The model under review builds one solid part; all positions refer to its coordinate system, in mm. Coordinates: 2 decimals unless noted, no trailing zeros. Write each loop counter-clockwise with the first axis right and the second up, starting at its lowest first coordinate (ties: lowest second). Pieces come first, ordered by that corner, then holes.
```python
from build123d import *

# Parameters (mm, degrees)
SKETCH_1_W           = 111
SKETCH_1_H           = 96
EXTRUDE_1_DEPTH      = 3
SKETCH_2_R           = 1.6
CUT_EXTRUDE_1_DEPTH  = 74.438749989
SKETCH_3_R           = 2.6
CUT_EXTRUDE_2_DEPTH  = 74.438749989
SKETCH_4_R           = 1.6
CUT_EXTRUDE_3_DEPTH  = 74.438749989
SKETCH_8_R           = 2.6
CUT_EXTRUDE_10_DEPTH = 74.438749989
SKETCH_5_W           = 18
SKETCH_5_H           = 50
CUT_EXTRUDE_4_DEPTH  = 74.438749989
FILLET_1_R           = 4
CUT_EXTRUDE_8_DEPTH  = 74.438749989
FILLET_2_R           = 2.5
CUT_EXTRUDE_9_DEPTH  = 74.438749989
FILLET_3_R           = 2.5


with BuildPart() as part:
    # 草图1 → 凸台-拉伸1 (new body)
    with BuildSketch(Plane.XY):
        Rectangle(SKETCH_1_W, SKETCH_1_H)
    extrude(amount=EXTRUDE_1_DEPTH)

    # 草图2 → 切除-拉伸1 (cut, through all)
    with BuildSketch(Plane.XY.offset(3)):
        with Locations((-50.5, -43)):
            Circle(SKETCH_2_R)
        with Locations((50.5, -43)):
            Circle(SKETCH_2_R)
    extrude(amount=-CUT_EXTRUDE_1_DEPTH, mode=Mode.SUBTRACT)

    # 草图3 → 切除-拉伸2 (cut, through all)
    with BuildSketch(Plane.XY.offset(3)):
        with Locations((-30, -43)):
            Circle(SKETCH_3_R)
        with Locations(Location((30, -43, 0), (0, 0, 180))):
            Circle(SKETCH_3_R)
    extrude(amount=-CUT_EXTRUDE_2_DEPTH, mode=Mode.SUBTRACT)

    # 草图4 → 切除-拉伸3 (cut, through all)
    with BuildSketch(Plane.XY.offset(3)):
        with Locations((-52.5, 18)):
            Circle(SKETCH_4_R)
        with Locations((-52.5, 38)):
            Circle(SKETCH_4_R)
        with Locations(Location((52.5, 38, 0), (0, 0, 180))):
            Circle(SKETCH_4_R)
        with Locations(Location((52.5, 18, 0), (0, 0, 180))):
            Circle(SKETCH_4_R)
    extrude(amount=-CUT_EXTRUDE_3_DEPTH, mode=Mode.SUBTRACT)

    # 草图8 → 切除-拉伸10 (cut, through all)
    with BuildSketch(Plane.XY.offset(3)):
        with Locations((-8, -32)):
            Circle(SKETCH_8_R)
        with Locations((-8, 33)):
            Circle(SKETCH_8_R)
    extrude(amount=-CUT_EXTRUDE_10_DEPTH, mode=Mode.SUBTRACT)

    # 草图5 → 切除-拉伸4 (cut, through all)
    with BuildSketch(Plane.XY.offset(3)):
        with Locations((-38, 0)):
            Rectangle(SKETCH_5_W, SKETCH_5_H)
        with Locations((38, 0)):
            Rectangle(SKETCH_5_W, SKETCH_5_H)
    extrude(amount=-CUT_EXTRUDE_4_DEPTH, mode=Mode.SUBTRACT)

    # 圆角1
    fillet_1_edges = [part.edges().sort_by_distance(p)[0] for p in [
        (-47, 25, 1.5),
        (-29, 25, 1.5),
        (-29, -25, 1.5),
        (-47, -25, 1.5),
        (47, -25, 1.5),
        (29, -25, 1.5),
        (29, 25, 1.5),
        (47, 25, 1.5),
    ]]
    fillet(fillet_1_edges, radius=FILLET_1_R)

    # 草图6 → 切除-拉伸8 (cut, through all)
    with BuildSketch(Plane.XY.offset(3)):
        with BuildLine():
            ThreePointArc((-3.753813954, 37.239092363), (-2.457683058, 30.70158252), (-8, 27))
            Line((-8, 27), (-8, 16.526279442))
            Line((-8, 16.526279442), (0, 2.669872981))
            Line((0, 2.669872981), (19.958548116, 37.239092363))
            Line((19.958548116, 37.239092363), (-3.753813954, 37.239092363))
        make_face()
        with BuildLine():
            Line((-8, -16.526279442), (-8, -26))
            ThreePointArc((-8, -26), (-2.193342004, -30.489131736), (-5.075634904, -37.239092363))
            Line((-5.075634904, -37.239092363), (19.958548116, -37.239092363))
            Line((19.958548116, -37.239092363), (0, -2.669872981))
            Line((0, -2.669872981), (-8, -16.526279442))
        make_face()
        Polygon((-2.5, 0), (-24, 37.239092363), (-24, -37.239092363), align=None)
        Polygon((24, -37.239092363), (24, 37.239092363), (2.5, 0), align=None)
    extrude(amount=-CUT_EXTRUDE_8_DEPTH, mode=Mode.SUBTRACT)

    # 圆角2
    fillet_2_edges = [part.edges().sort_by_distance(p)[0] for p in [
        (24, -37.239092363, 1.5),
        (2.5, 0, 1.5),
        (24, 37.239092363, 1.5),
        (-8, 27, 1.5),
        (-3.753813954, 37.239092363, 1.5),
        (19.958548116, 37.239092363, 1.5),
        (0, 2.669872981, 1.5),
        (-8, 16.526279442, 1.5),
        (-5.075634904, -37.239092363, 1.5),
        (-8, -26, 1.5),
        (-8, -16.526279442, 1.5),
        (0, -2.669872981, 1.5),
        (19.958548116, -37.239092363, 1.5),
        (-24, -37.239092363, 1.5),
        (-24, 37.239092363, 1.5),
        (-2.5, 0, 1.5),
    ]]
    fillet(fillet_2_edges, radius=FILLET_2_R)

    # 草图7 → 切除-拉伸9 (cut, through all)
    with BuildSketch(Plane.XY.offset(3)):
        Polygon((-19.172154979, 42), (-47.5, 42), (-47.5, 38), (-47.5, 28.5), (-30.5, 28.5), align=None)
        Polygon((-47.5, -36), (-47.5, -28.5), (-31.5, -28.5), (-25.5, -36), align=None)
        Polygon((25.5, -36), (47.5, -36), (47.5, -28.5), (31.5, -28.5), align=None)
        Polygon((47.5, 42), (47.5, 38), (47.5, 28.5), (30.5, 28.5), (19.172154979, 42), align=None)
    extrude(amount=-CUT_EXTRUDE_9_DEPTH, mode=Mode.SUBTRACT)

    # 圆角3
    fillet_3_edges = [part.edges().sort_by_distance(p)[0] for p in [
        (47.5, 42, 1.5),
        (47.5, 28.5, 1.5),
        (30.5, 28.5, 1.5),
        (19.172154979, 42, 1.5),
        (47.5, -36, 1.5),
        (25.5, -36, 1.5),
        (31.5, -28.5, 1.5),
        (47.5, -28.5, 1.5),
        (-47.5, -36, 1.5),
        (-47.5, -28.5, 1.5),
        (-31.5, -28.5, 1.5),
        (-25.5, -36, 1.5),
        (-47.5, 42, 1.5),
        (-19.172154979, 42, 1.5),
        (-30.5, 28.5, 1.5),
        (-47.5, 28.5, 1.5),
    ]]
    fillet(fillet_3_edges, radius=FILLET_3_R)


solid = part.part
```
Item 1: Take a section at B-B, the plane z = 0.85. Count the separate pieces of the cut face and the enclosed holes in it, plus the area to 3 significant figures.
Solved:
separate pieces: 1
enclosed holes: 20
area: 5,350 mm2
Item 2: For pin 1 (2.5 mm diameter, centred on x = -52.5, y = 18, fed in from +Z), flat-tipped, find the tip position at first contact; note if it passes through.
Solved:
pin 1: passes through
Item 3: To check wall thickness, follow line 1 along Y through (x, z) = (-36.5, 1.55); line 2 along Y through (x, z) = (52.5, 2.1); line 3 along X through (y, z) = (29, 1.35). State the ranges of each line that lie inside material, in increasing order.
Solved:
line 1: y = -48 to -36, -28.5 to -25, 25 to 28.5, 42 to 48
line 2: y = -48 to 16.4, 19.6 to 36.4, 39.6 to 48
line 3: x = -55.5 to -46.5, -30.17 to -23.75, -19.24 to -3.53, 15.2 to 19.24, 23.75 to 30.17, 46.5 to 55.5
Item 4: Mouldability with a two-part tool opening along Y and no side actions: class faces 1 (the face through (-2.801, 30.004, 1.521)), 2 (the face through (-1, 48, 1)), 3 (the face through (-4.88, -11.12, 1.52)) as pulls with the +Y half, pulls with the -Y half, needs draft (parallel to the pull), parting line crosses it, or undercut.
Solved:
face 1: undercut
face 2: pulls with the +Y half
face 3: undercut
Item 5: Take a section at A-A, the plane x = 11.5. Write out the cut boundary in (y, z), plus the area to 3 significant figures.
Solved:
outline: (-48, 0) - (-37.24, 0) - (-37.24, 3) - (-48, 3) - close; (-22.59, 0) - (-15.59, 0) - (-15.59, 3) - (-22.59, 3) - close; (15.59, 0) - (22.59, 0) - (22.59, 3) - (15.59, 3) - close; (37.24, 0) - (48, 0) - (48, 3) - (37.24, 3) - close
area: 107 mm2
